from build123d import *

# Parameters (mm, degrees)
SKETCH2_W           = 12.7
SKETCH2_H           = 12.7
BOSS_EXTRUDE1_DEPTH = 40.64
FILLET1_R           = 6.35
SKETCH3_W           = 12.7
SKETCH3_H           = 12.7
CUT_EXTRUDE2_DEPTH  = 42.620362805


with BuildPart() as part:
    # Sketch2 → Boss-Extrude1 (new body)
    with BuildSketch(Plane(origin=(0, 0, 0), x_dir=(0, 0, -1), z_dir=(1, 0, 0))):
        Rectangle(SKETCH2_W, SKETCH2_H)
    extrude(amount=BOSS_EXTRUDE1_DEPTH)

    # Fillet1
    fillet1_edges = [part.edges().sort_by_distance(p)[0] for p in [
        (40.64, 0, 6.35),
    ]]
    fillet(fillet1_edges, radius=FILLET1_R)

    # Sketch3 → Cut-Extrude2 (cut, through all)
    with BuildSketch(Plane.ZY):
        Rectangle(SKETCH3_W, SKETCH3_H)
        with BuildLine():
            ThreePointArc((2.488681579, 0), (3.278329429, -1.162432523), (3.556, -2.54))
            ThreePointArc((3.556, -2.54), (-1.377567477, -5.818329429), (-2.488681579, 0))
            ThreePointArc((-2.488681579, 0), (-1.377567477, 5.818329429), (3.556, 2.54))
            ThreePointArc((3.556, 2.54), (3.278329429, 1.162432523), (2.488681579, 0))
        make_face(mode=Mode.SUBTRACT)
    extrude(amount=-CUT_EXTRUDE2_DEPTH, mode=Mode.SUBTRACT)


solid = part.part
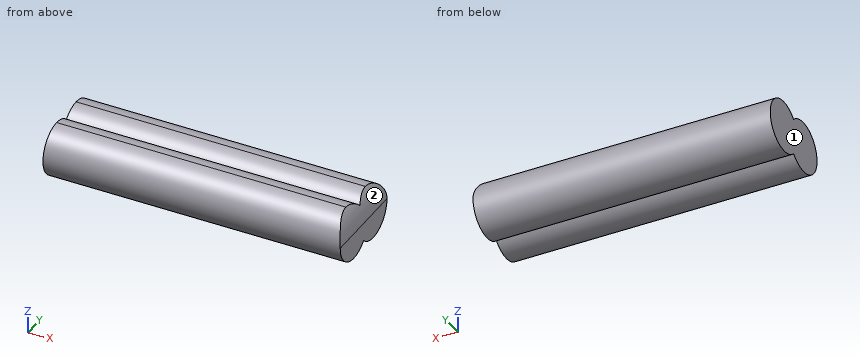
Check sheet for the modelled part. Datum: model origin and axes. Units: mm. Face numbers are marked on the shaded views. Coordinates: 2 decimals unless noted, no trailing zeros. Loops run counter-clockwise (first coordinate to the right, second up) from the corner with the lowest first, then second, coordinate; pieces in that order, holes last. Notation, with made-up numbers: (22.5, -39) -> (60.5, -39) arc R27 cw to (60.5, -1) -> close; hole circle Ø5 at (18, 6). An arc over 180 degrees is marked (long way). Write item = value, one per line. Start each with the question number.
1. Section check B-B on x = 20.5. Record the cut outline in (y, z).
2. Section check C-C on z = 1.75. Record the cut outline in (x, y).
3. Material ranges on line 1 (Z direction, x = 24, y = 2.75); line 2 (Y direction, x = 20, z = -3); line 3 (Z direction, x = 31, y = 1), recorded low to high.
4. Draft check along X on the marked faces 1 and 2. Enter one of: released by +X, released by -X, zero draft, split by the parting line, or undercut.
5. Depth check by flat-ended pin: P1, Ø1, axis at x = 29, y = -0.5, coming from the +Z side; P2, Ø2, axis at x = 17.5, y = -4, coming from the +Z side; P3, Ø2, axis at x = 21.5, z = 2.5, coming from the -Y side. Enter the tip coordinate at first touch or a pass-through.
6. Section check A-A on y = -5. Record the cut outline in (x, z), then the cut area to 3 significant figures.
Responses:
q1.outline = (0, -2.49) arc R3.56 ccw (long way) to (0, 2.49) arc R3.56 ccw (long way) to start
q2.outline = (0, -5.64) -> (40.39, -5.64) -> (40.39, 5.64) -> (0, 5.64) -> close
q3.line_1 = -3.55 to 3.55
q3.line_2 = -4.45 to -0.63, 0.63 to 4.45
q3.line_3 = -3.21 to 3.21
q4.face_1 = released by -X
q4.face_2 = released by +X
q5.P1 = 3.21
q5.P2 = 3.53
q5.P3 = -5.76
q6.outline = (0, -2.57) -> (40.64, -2.57) -> (40.64, 0) arc R6.35 ccw to (40.1, 2.57) -> (0, 2.57) -> close
q6.area = 208 mm2
